from build123d import *

# Parameters (mm, degrees)
CROQUIS1_R              = 3.5
CROQUIS1_R_2            = 15
CROQUIS1_W              = 26
CROQUIS1_H              = 76.5
CROQUIS1_H_2            = 13
CROQUIS1_W_2            = 13
CROQUIS1_H_3            = 26
SALIENTE_EXTRUIR1_DEPTH = 19


with BuildPart() as part:
    # Croquis1 → Saliente-Extruir1 (new body)
    with BuildSketch(Plane.XY):
        Polygon((-301, 194), (-301, 175), (301, 175), (301, 194), (401, 194), (431, 164), (431, 30), (401, 0), (250, 0), (250, 25), (-250, 25), (-250, 0), (-401, 0), (-431, 30), (-431, 164), (-401, 194), align=None)
        with Locations((-391, 97)):
            Circle(CROQUIS1_R, mode=Mode.SUBTRACT)
        with Locations((391, 97)):
            Circle(CROQUIS1_R, mode=Mode.SUBTRACT)
        with Locations((0, 100)):
            Circle(CROQUIS1_R_2, mode=Mode.SUBTRACT)
        with Locations((-25, 125)):
            Circle(CROQUIS1_R, mode=Mode.SUBTRACT)
        with Locations((25, 125)):
            Circle(CROQUIS1_R, mode=Mode.SUBTRACT)
        with Locations((25, 75)):
            Circle(CROQUIS1_R, mode=Mode.SUBTRACT)
        with Locations((-25, 75)):
            Circle(CROQUIS1_R, mode=Mode.SUBTRACT)
        with Locations((-298, 116.75)):
            Rectangle(CROQUIS1_W, CROQUIS1_H, mode=Mode.SUBTRACT)
        with Locations((298, 116.75)):
            Rectangle(CROQUIS1_W, CROQUIS1_H, mode=Mode.SUBTRACT)
        with Locations((378, 26.5)):
            Rectangle(CROQUIS1_W, CROQUIS1_H_2, mode=Mode.SUBTRACT)
        with Locations((-378, 26.5)):
            Rectangle(CROQUIS1_W, CROQUIS1_H_2, mode=Mode.SUBTRACT)
        with Locations((391, 155)):
            Rectangle(CROQUIS1_W_2, CROQUIS1_H_3, mode=Mode.SUBTRACT)
        with Locations((-391, 155)):
            Rectangle(CROQUIS1_W_2, CROQUIS1_H_3, mode=Mode.SUBTRACT)
    extrude(amount=SALIENTE_EXTRUIR1_DEPTH)


solid = part.part
The model under review builds one solid part; all positions refer to its coordinate system, in mm. A direction names the side the tool comes from. Round coordinates to 2 decimals unless told otherwise and drop trailing zeros. Write each loop counter-clockwise with the first axis right and the second up, starting at its lowest first coordinate (ties: lowest second). Pieces come first, ordered by that corner, then holes. Notation, with made-up numbers: (-10.75, 38) -> (47.25, 38) arc R19 ccw to (47.25, 63) -> close; hole circle Ø9 at (-21, 87.25). An arc over 180 degrees is marked (long way). Answer as a JSON object with one key per item and string values.
1. To check wall thickness, follow line 1 along X through (y, z) = (149.5, 13.25); line 2 along Y through (x, z) = (-25, 12.25); line 3 along X through (y, z) = (102, 16). State the ranges of each line that lie inside material, in increasing order.
Results found:
{"line 1": "x = -431 to -397.5, -384.5 to -311, -285 to 285, 311 to 384.5, 397.5 to 431", "line 2": "y = 25 to 71.5, 78.5 to 121.5, 128.5 to 175", "line 3": "x = -431 to -311, -285 to -14.87, 14.87 to 285, 311 to 431"}
2. We need section A-A on z = 11.75. State how many separate pieces and enclosed holes the cut face has, and give its area (3 significant figures).
Results found:
{"separate pieces": "1", "enclosed holes": "13", "area": "135,000 mm^2"}
3. The part is to be moulded in two halves that separate along Y. For faces 1 (the face through (-324, 0, 9)), 2 (the face through (416, 179, 9)), 3 (the face through (-250, 13, 9)), 4 (the face through (378, 20, 9)), say which applies: pulls with the +Y half, pulls with the -Y half, needs draft (parallel to the pull), parting line crosses it, or undercut.
Results found:
{"face 1": "pulls with the -Y half", "face 2": "pulls with the +Y half", "face 3": "needs draft", "face 4": "undercut"}
4. We need section B-B on x = 46.5. State the section outline as (y, z) points.
Results found:
{"outline": "(25, 0) -> (175, 0) -> (175, 19) -> (25, 19) -> close"}
5. Machinability: for faces 5 (the face through (-431, 96, 9)), 6 (the face through (431, 98, 9)), 7 (the face through (301, 184, 9)), 8 (the face through (250, 12, 9)), 9 (the face through (285, 116, 9)), which of the approach directions +Z, -Z, +X, -X, +Y, -Y give a long, thin tool a straight path to every point of the face, cutting with its end or side? Answer none if there is none.
Results found:
{"face 5": "+Z, -Z, -X, +Y, -Y", "face 6": "+Z, -Z, +X, +Y, -Y", "face 7": "+Z, -Z, +Y", "face 8": "+Z, -Z, -Y", "face 9": "+Z, -Z"}
6. Clearance check with flat-ended pins moving along their axes: pin 1 (9.5 mm diameter, centred on x = -293, z = 6, fed in from +Y); pin 2 (5.5 mm diameter, centred on y = 186.5, z = 7, fed in from -X). State where each tip first meets the part, or that it passes through.
Results found:
{"pin 1": "stops at y = 175", "pin 2": "stops at x = -411.25"}
